Autodesk Fusion 360 part; units mm, degrees
sketch "Sketch1" plane through (0, 0, 0) normal (0, 1, 0) x (1, 0, 0)
  line L0 (0, 0) -> (15.5, 0)
  line L1 (15.5, 0) -> (15.5, -12.5)
  line L2 (15.5, -12.5) -> (0, -12.5)
  line L3 (0, -12.5) -> (0, 0)
  line L4 (2, -2) -> (13.5, -2)
  line L5 (13.5, -2) -> (13.5, -10.5)
  line L6 (13.5, -10.5) -> (2, -10.5)
  line L7 (2, -10.5) -> (2, -2)
  dimension "d1" = 15.5
  dimension "d2" = 12.5
  dimension "d3" = 2
extrude "Extrude1" add sketch "Sketch1" along normal blind 18
extrude "Extrude2" add sketch "Sketch1" along normal blind 3 contours L4 L5 L6 L7
sketch "Sketch2" plane through (0, 0, 0) normal (0, 0, -1) x (1, 0, 0)
  line L0 (15.5, 0) -> (0, 0)
  line L1 (0, 0) -> (0, -18)
  line L2 (0, -18) -> (15.5, -18)
  line L3 (15.5, -18) -> (15.5, 0)
  line L4 (0, -18) -> (0, -7)
  line L5 (0, -7) -> (15.5, -7)
  line L6 (15.5, -7) -> (15.5, -18)
  circle A0 centre (14.15, -8.35) radius 1.35
  circle A1 centre (1.35, -8.35) radius 1.35
  dimension "d8" = 11
  dimension "d9" = 1.35
  dimension "d10" = 1.35
extrude "Extrude3" add sketch "Sketch2" along normal blind 2 contours A0 | A1
equation "d9 = ( 2.7 / 2 ) * 1 mm"
equation "d10 = ( 2.7 / 2 ) * 1 mm"
Here's how the part is built. I have some questions about the finished solid (model axes, mm). A direction names the side the tool comes from. Coordinates: 2 decimals unless noted, no trailing zeros. Write each loop counter-clockwise with the first axis right and the second up, starting at its lowest first coordinate (ties: lowest second). Pieces come first, ordered by that corner, then holes. Notation, with made-up numbers: (53.25, 47.5) -> (74.25, 47.5) arc R13 cw to (74.25, 65.5) -> close; hole circle Ø6 at (-16, 37). An arc over 180 degrees is marked (long way). Use a Markdown table: item, result. Add a question column.
(1) For faces 1 (the cylindrical face through (1.174, 9.689, -0.986)), 2 (the flat face through (14, 8, -2)), 3 (the flat face through (13.5, 10, 6)), which set-ups out of +Z, -Z, +X, -X, +Y, -Y let a thin tool reach every point of the face, with its end or its side?
(2) If we section it at B-B, the plane x = 11.25: Write out the boundary of the cut face in (y, z), and give its area (3 significant figures).
(3) I'm going to push flat-ended pins straight in: P1, Ø4, axis at x = 12.5, y = 10.5, coming from the -Z side; P2, Ø4.5, axis at x = 9, y = 10, coming from the -Z side; P3, Ø2.5, axis at x = 9, z = 4.5, coming from the +Y side. Where does each tip first touch, or does it pass through?
(4) Please list where these lines run through material, in increasing order: line 1 (X direction, y = 15.25, z = 4.75); line 2 (Z direction, x = 12, y = 8); line 3 (Z direction, x = 13.25, y = 9.25).
(5) If we section it at C-C, the plane z = 2.5: Write out the boundary of the cut face in (x, y), and give its area (4 significant figures).
(6) We'd pull the mould along X, two halves only. Please class faces 4 (the flat face through (8, 18, 1)), 5 (the flat face through (8, 10, 10.5)), 6 (the flat face through (15.5, 9, 6)): +X half, -X half, draft (parallel to the pull), parting line (faces both ways), or undercut.
(7) If we section it at A-A, the plane y = 15.5: Write out the boundary of the cut face in (x, z), and give its area (3 significant figures).
Outcome:
| question | item | result |
|---|---|---|
| 1 | face 1 | -Z |
| 1 | face 2 | -Z, +X, -X, +Y, -Y |
| 1 | face 3 | +Y |
| 2 | outline | (0, 0) -> (18, 0) -> (18, 2) -> (3, 2) -> (3, 10.5) -> (18, 10.5) -> (18, 12.5) -> (0, 12.5) -> close |
| 2 | area | 97.5 mm^2 |
| 3 | P1 | stops at z = -2 |
| 3 | P2 | stops at z = 0 |
| 3 | P3 | stops at y = 3 |
| 4 | line 1 | x = 0 to 2, 13.5 to 15.5 |
| 4 | line 2 | z = 0 to 2, 10.5 to 12.5 |
| 4 | line 3 | z = -2 to 2, 10.5 to 12.5 |
| 5 | outline | (0, 0) -> (15.5, 0) -> (15.5, 18) -> (13.5, 18) -> (13.5, 3) -> (2, 3) -> (2, 18) -> (0, 18) -> close |
| 5 | area | 106.5 mm^2 |
| 6 | face 4 | draft |
| 6 | face 5 | undercut |
| 6 | face 6 | +X half |
| 7 | outline | (0, 0) -> (15.5, 0) -> (15.5, 12.5) -> (0, 12.5) -> close; hole (2, 2) -> (13.5, 2) -> (13.5, 10.5) -> (2, 10.5) -> close |
| 7 | area | 96.0 mm^2 |
